Study the drawing (mm; zero at the part's minimum x, y, z) and answer. Coordinates: 2 decimals unless noted, no trailing zeros. Order: outer loops, then holes, each group sorted by start corner. A loop starts at its lowest first (then second) coordinate and runs counter-clockwise, first axis right, second up. Notation, with made-up numbers: M 5.5,-26 L 21.5,-26 A16 ccw 21.5,-11 Z; hole C 4.5,18.25 d1. An arc over 180 degrees is marked long. Put each result on its own line as item: value.
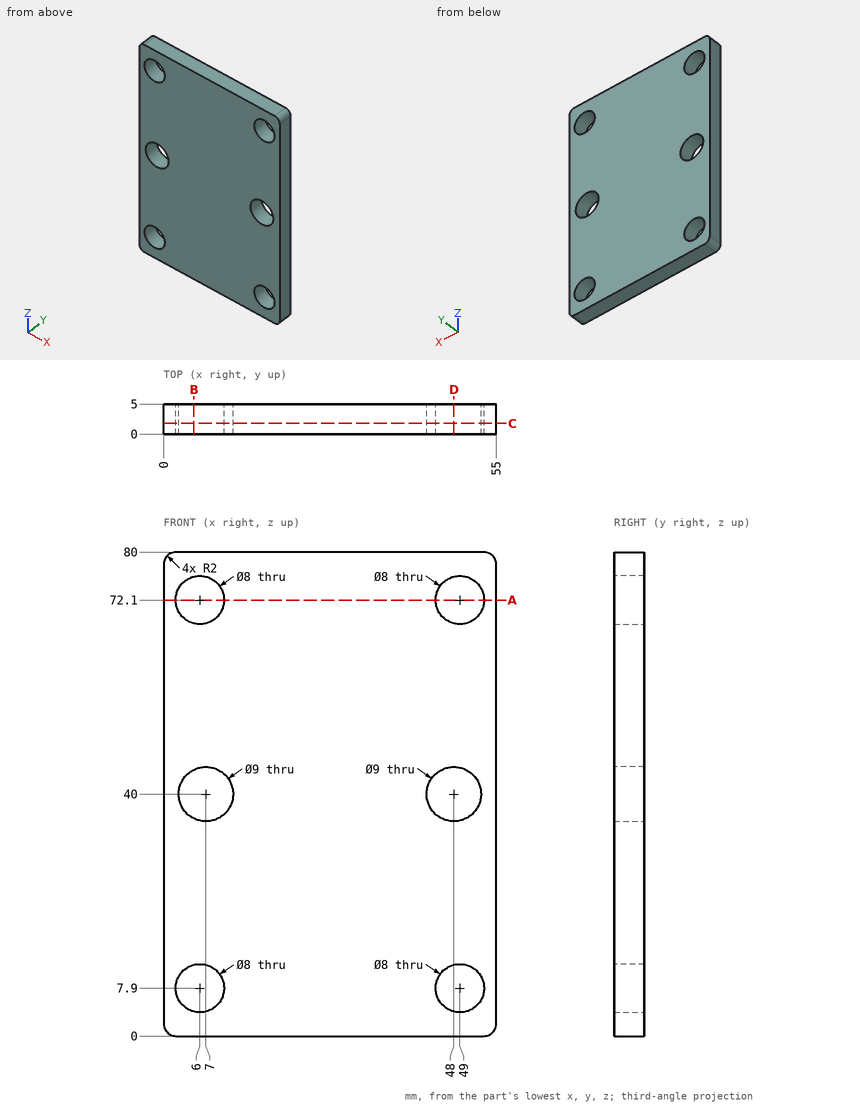
Q1. Find section C-C on y = 1.8. Write down the section's boundary in (x, z).
Answers below:
outline: M 0,2 A2 ccw 2,0 L 53,0 A2 ccw 55,2 L 55,78 A2 ccw 53,80 L 2,80 A2 ccw 0,78 Z; hole C 6,7.9 d8; hole C 6,72.1 d8; hole C 7,40 d9; hole C 48,40 d9; hole C 49,7.9 d8; hole C 49,72.1 d8
Q2. Given pin 1 (7 mm diameter, centred on x = 49, z = 72.1, fed in from -Y); pin 2 (3 mm diameter, centred on y = 2, z = 21, fed in from -X), each flat-ended and moving along its own axis, determine where each tip first touches the part or whether it passes through.
Answers below:
pin 1: passes through
pin 2: stops at x = 0
Q3. Find section B-B on x = 5. Write down the section's boundary in (y, z), plus the area to 3 significant figures.
Answers below:
outline: M 0,0 L 5,0 L 5,4.03 L 0,4.03 Z; M 0,11.77 L 5,11.77 L 5,35.97 L 0,35.97 Z; M 0,44.03 L 5,44.03 L 5,68.23 L 0,68.23 Z; M 0,75.97 L 5,75.97 L 5,80 L 0,80 Z
area: 282 mm^2
Q4. Find section D-D on x = 48. Write down the section's boundary in (y, z).
Answers below:
outline: M 0,0 L 5,0 L 5,4.03 L 0,4.03 Z; M 0,11.77 L 5,11.77 L 5,35.5 L 0,35.5 Z; M 0,44.5 L 5,44.5 L 5,68.23 L 0,68.23 Z; M 0,75.97 L 5,75.97 L 5,80 L 0,80 Z
Q5. Find section A-A on z = 72.1. Write down the section's boundary in (x, y).
Answers below:
outline: M 0,0 L 2,0 L 2,5 L 0,5 Z; M 10,0 L 45,0 L 45,5 L 10,5 Z; M 53,0 L 55,0 L 55,5 L 53,5 Z
Q6. Consider line 1 along X through (y, z) = (1.8, 40); line 2 along X through (y, z) = (2.6, 7.9); line 3 along Z through (x, y) = (49.5, 3.05). Determine where each line is inside the solid, lowest interval first.
Answers below:
line 1: x = 0 to 2.5, 11.5 to 43.5, 52.5 to 55
line 2: x = 0 to 2, 10 to 45, 53 to 55
line 3: z = 0 to 3.93, 11.87 to 35.76, 44.24 to 68.13, 76.07 to 80
